For this review, take the finished solid that the model builds, in its own axes (mm). A direction names the side the tool comes from. Coordinates: 2 decimals unless noted, no trailing zeros. Loops run counter-clockwise (first coordinate to the right, second up) from the corner with the lowest first, then second, coordinate; pieces in that order, holes last. Notation, with made-up numbers: (-6, 64) - (27, 64) arc R19 cw to (27, 78) - close; hole circle Ø6 at (-34.75, -33.5). An arc over 180 degrees is marked (long way). Use one line per item in the form item = value. Start each with the question number.
1. Add section A-A on x = 22.5. Give the boundary of the cut face in (y, z) (3 decimals), and give its area (3 significant figures).
2. Add section B-B on z = 28. Give the boundary of the cut face in (x, y) (3 decimals), and give its area (3 significant figures).
3. Machinability: for faces 4 (the face through (-1, 3.175, -1)), 5 (the face through (-38, 0, -1.899)), 6 (the face through (-41, 0, 3.969)), which of the approach directions +Z, -Z, +X, -X, +Y, -Y give a long, thin tool a straight path to every point of the face, cutting with its end or side? Answer none if there is none.
4. For pin 1 Ø3.5 at (x, z) = (-22.5, 28) entering from -Y; pin 2 Ø2 at (y, z) = (1, -4.5) entering from -X (3 decimals), all flat-tipped, find the tip position at first contact; note any pin that passes through.
5. Draft analysis for pull direction Z (two halves, no side actions). For faces 1 (the face through (-50, 0, -6.35)), 2 (the face through (-1, -3.175, -1)), 3 (the face through (-1, 0, 57.15)), state which applies: +Z half, -Z half, draft (parallel to the pull), parting line (faces both ways), or undercut.
6. Add section D-D on x = -22.5. Give the boundary of the cut face in (y, z) (3 decimals).
7. Add section C-C on z = -50.8. Give the boundary of the cut face in (x, y) (3 decimals), and give its area (3 significant figures).
8. To check wall thickness, follow probe 1 along Z at (x, y) = (-22.5, 0.75); probe 2 along X at (y, z) = (-1.5, 2.5) (3 decimals); probe 3 along Z at (x, y) = (-43, 1). State the ranges of each line that lie inside material, in increasing order.
```python
from build123d import *

# Parameters (mm, degrees)
SKETCH1_W                      = 105.41
SKETCH1_H                      = 114.3
BOSS_EXTRUDE1_DEPTH            = 3.175
F_4_0_4_DIAMETER_HOLE1_D       = 4
LPATTERN1_COUNT                = 2
LPATTERN1_PITCH                = 56
LPATTERN1_COUNT_DIR2           = 2
LPATTERN1_PITCH_DIR2           = 45
F_8_CLEARANCE_HOLE1_D          = 4.4958
MIRROR2_COPY_1_D               = 4.4958
F_6_CLEARANCE_HOLE1_AT_2_COUNT = 2
F_6_CLEARANCE_HOLE1_AT_2_PITCH = 28.575
CUT_EXTRUDE1_REACH             = 80.002


with BuildPart() as part:
    # Sketch1 → Boss-Extrude1 (new, symmetric)
    with BuildSketch(Plane(origin=(0, 0, 0), x_dir=(1, 0, 0), z_dir=(0, 1, 0))):
        Rectangle(SKETCH1_W, SKETCH1_H)
    extrude(amount=BOSS_EXTRUDE1_DEPTH, both=True)

    # Ø4.0 (4) Diameter Hole1 (through all)
    with Locations(Plane(origin=(0, 3.175, 0), x_dir=(1, 0, 0), z_dir=(0, 1, 0))):
        with Locations((22.5, 28)):
            f_4_0_4_diameter_hole1 = Hole(F_4_0_4_DIAMETER_HOLE1_D / 2)

    # LPattern1: 4.0 _4_ Diameter Hole1 2 × 2
    with Locations(*[(-j * LPATTERN1_PITCH_DIR2, 0, i * LPATTERN1_PITCH) for i in range(LPATTERN1_COUNT) for j in range(LPATTERN1_COUNT_DIR2) if (i, j) != (0, 0)]):
        add(f_4_0_4_diameter_hole1, mode=Mode.SUBTRACT)

    # #8 Clearance Hole1 (through all)
    with Locations(Plane(origin=(0, 3.175, 0), x_dir=(1, 0, 0), z_dir=(0, 1, 0))):
        with Locations((-46.355, 50.8)):
            f_8_clearance_hole1 = Hole(F_8_CLEARANCE_HOLE1_D / 2)

    # Mirror1: #8 Clearance Hole1 across plane
    add(f_8_clearance_hole1.mirror(Plane.XY), mode=Mode.SUBTRACT)

    # Mirror2: #8 Clearance Hole1 across plane
    add(f_8_clearance_hole1.mirror(Plane(origin=(0, 0, 0), x_dir=(0, 0, 1), z_dir=(1, 0, 0))), mode=Mode.SUBTRACT)

    # Mirror2 copy 1 (through all)
    with Locations(Plane(origin=(0, 3.175, 0), x_dir=(-1, 0, 0), z_dir=(0, 1, 0))):
        with Locations((-46.355, 50.8)):
            Hole(MIRROR2_COPY_1_D / 2)

    # Sketch6 → #6 Clearance Hole1 (revolve, cut)
    with BuildSketch(Plane(origin=(22.5, 3.175, -50.8), x_dir=(0, 0, 1), z_dir=(1, 0, 0))):
        Polygon((0, 0), (0, 7.403068321), (1.7526, 6.35), (1.7526, 0), align=None)
    f_6_clearance_hole1 = revolve(axis=Axis((22.5, 9.525, -50.8), (0, -1, 0)), mode=Mode.SUBTRACT)

    # #6 Clearance Hole1 at 2: #6 Clearance Hole1 ×2
    with Locations(*[(-i * F_6_CLEARANCE_HOLE1_AT_2_PITCH, 0, 0) for i in range(1, F_6_CLEARANCE_HOLE1_AT_2_COUNT)]):
        add(f_6_clearance_hole1, mode=Mode.SUBTRACT)

    # Sketch8 → Cut-Extrude1 (cut, up to next)
    with BuildSketch(Plane(origin=(0, 3.175, 0), x_dir=(1, 0, 0), z_dir=(0, 1, 0)), mode=Mode.PRIVATE) as cut_extrude1_sk1:
        Polygon((-52.705, -6.35), (-52.705, 6.35), (-46.355, 6.35), (-46.355, 1.89865), (-42.8545625, 1.89865), (-42.8545625, 3.96875), (-40.0764375, 3.96875), (-40.0764375, 1.89865), (-36.576, 1.89865), (-36.576, -1.89865), (-40.0764375, -1.89865), (-40.0764375, -3.96875), (-42.8545625, -3.96875), (-42.8545625, -1.89865), (-46.355, -1.89865), (-46.355, -6.35), align=None)
    cut_extrude1_tool1 = extrude(cut_extrude1_sk1.sketch, amount=-CUT_EXTRUDE1_REACH, mode=Mode.PRIVATE) & part.part
    add(cut_extrude1_tool1.solids().sort_by_distance((-46.496113, 3.175, 0))[0], mode=Mode.SUBTRACT)

    # Mirror3: #6 Clearance Hole1 across plane
    add(f_6_clearance_hole1.mirror(Plane.XY), mode=Mode.SUBTRACT)

    # Mirror3 copy 1 sketch → Mirror3 copy 1 (revolve, cut)
    with BuildSketch(Plane(origin=(-6.075, 3.175, 50.8), x_dir=(0, 0, -1), z_dir=(1, 0, 0))):
        Polygon((0, 0), (0, -7.403068321), (1.7526, -6.35), (1.7526, 0), align=None)
    revolve(axis=Axis((-6.075, 9.525, 50.8), (0, 1, 0)), mode=Mode.SUBTRACT)


solid = part.part
```
Conclusion:
q1.outline = (-3.175, -57.15) - (3.175, -57.15) - (3.175, -52.553) - (-3.175, -52.553) - close; (-3.175, -49.047) - (3.175, -49.047) - (3.175, -30) - (-3.175, -30) - close; (-3.175, -26) - (3.175, -26) - (3.175, 26) - (-3.175, 26) - close; (-3.175, 30) - (3.175, 30) - (3.175, 49.047) - (-3.175, 49.047) - close; (-3.175, 52.553) - (3.175, 52.553) - (3.175, 57.15) - (-3.175, 57.15) - close
q1.area = 630 mm^2
q2.outline = (-52.705, -3.175) - (-24.5, -3.175) - (-24.5, 3.175) - (-52.705, 3.175) - close; (-20.5, -3.175) - (20.5, -3.175) - (20.5, 3.175) - (-20.5, 3.175) - close; (24.5, -3.175) - (52.705, -3.175) - (52.705, 3.175) - (24.5, 3.175) - close
q2.area = 619 mm^2
q3.face_4 = +Z, -Z, +X, -X, +Y
q3.face_5 = -X, +Y, -Y
q3.face_6 = +Y, -Y
q4.pin_1 = through
q4.pin_2 = -46.355
q5.face_1 = undercut
q5.face_2 = draft
q5.face_3 = +Z half
q6.outline = (-3.175, -57.15) - (3.175, -57.15) - (3.175, -30) - (-3.175, -30) - close; (-3.175, -26) - (3.175, -26) - (3.175, 26) - (-3.175, 26) - close; (-3.175, 30) - (3.175, 30) - (3.175, 57.15) - (-3.175, 57.15) - close
q7.outline = (-52.705, -3.175) - (-48.603, -3.175) - (-48.603, 3.175) - (-52.705, 3.175) - close; (-44.107, -3.175) - (-7.828, -3.175) - (-7.828, 3.175) - (-44.107, 3.175) - close; (-4.322, -3.175) - (20.747, -3.175) - (20.747, 3.175) - (-4.322, 3.175) - close; (24.253, -3.175) - (44.107, -3.175) - (44.107, 3.175) - (24.253, 3.175) - close; (48.603, -3.175) - (52.705, -3.175) - (52.705, 3.175) - (48.603, 3.175) - close
q7.area = 568 mm^2
q8.probe_1 = -57.15 to -30, -26 to 26, 30 to 57.15
q8.probe_2 = -46.355 to -42.855, -40.076 to 52.705
q8.probe_3 = -57.15 to -1.9, 1.9 to 57.15
